Here's how the part is built. I have some questions about the finished solid (model axes, mm). Face numbers are marked on the shaded views. Round coordinates to 2 decimals unless told otherwise and drop trailing zeros. Write each loop counter-clockwise with the first axis right and the second up, starting at its lowest first coordinate (ties: lowest second). Pieces come first, ordered by that corner, then holes. Notation, with made-up numbers: (16, -2.5) -> (43, -2.5) arc R21 ccw to (43, 22.5) -> close; hole circle Ø4 at (34, 87.5). An arc over 180 degrees is marked (long way). Answer in a Markdown table with one row per item.
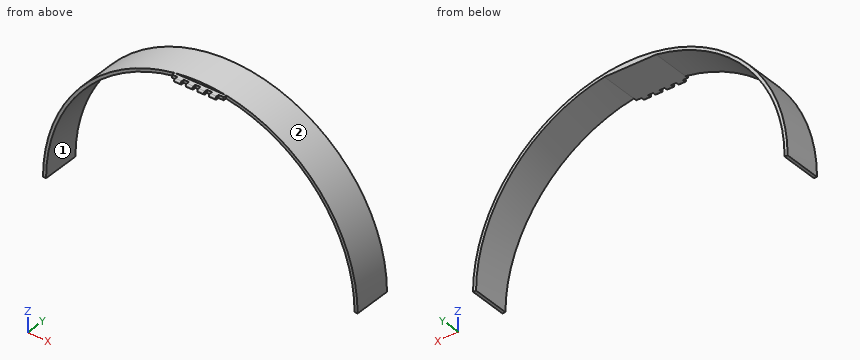
from build123d import *

# Parameters (mm, degrees)
SKETCH1_W              = 50
SKETCH1_H              = 3
BOSS_EXTRUDE1_DEPTH    = 40
SKETCH2_W              = 6.25
SKETCH2_H              = 3
BOSS_EXTRUDE2_DEPTH    = 4
FILLET1_R              = 1.5
LPATTERN1_COUNT        = 4
LPATTERN1_PITCH        = 11.25
FILLET1_OF_LPATTERN1_R = 1.5
SKETCH3_W              = 3
SKETCH3_H              = 37
SKETCH8_R              = 0.75
CUT_EXTRUDE1_DEPTH     = 232.430553417
CUT_EXTRUDE2_DEPTH     = 218.721568988


with BuildPart() as part:
    # Sketch1 → Boss-Extrude1 (new body)
    with BuildSketch(Plane(origin=(0, 0, 0), x_dir=(1, 0, 0), z_dir=(0, 1, 0))):
        Rectangle(SKETCH1_W, SKETCH1_H)
    extrude(amount=BOSS_EXTRUDE1_DEPTH)

    # Sketch2 → Boss-Extrude2 (add)
    with BuildSketch(Plane.XZ):
        with Locations((-16.875, 0)):
            Rectangle(SKETCH2_W, SKETCH2_H)
    boss_extrude2 = extrude(amount=BOSS_EXTRUDE2_DEPTH)

    # Fillet1
    fillet1_edges = [part.edges().sort_by_distance(p)[0] for p in [
        (-16.875, -4, 1.5),
        (-16.875, -4, -1.5),
    ]]
    fillet(fillet1_edges, radius=FILLET1_R - 0.0001)  # a hair under: the kernel refuses the full size

    # LPattern1: Boss-Extrude2 ×4
    with Locations(*[(i * LPATTERN1_PITCH, 0, 0) for i in range(1, LPATTERN1_COUNT)]):
        add(boss_extrude2)

    # Fillet1 of LPattern1
    fillet1_of_lpattern1_edges = [part.edges().sort_by_distance(p)[0] for p in [
        (-5.625, -4, 1.5),
        (-5.625, -4, -1.5),
        (5.625, -4, 1.5),
        (5.625, -4, -1.5),
        (16.875, -4, 1.5),
        (16.875, -4, -1.5),
    ]]
    fillet(fillet1_of_lpattern1_edges, radius=FILLET1_OF_LPATTERN1_R - 0.0001)  # a hair under: the kernel refuses the full size

    # Sweep2: sweep along a path in Sketch7
    with BuildLine(Plane(origin=(0, 38.5, 0), x_dir=(1, 0, 0), z_dir=(0, 1, 0))) as sweep2_path:
        ThreePointArc((-149.86, 148.775138892), (0, -1.084861108), (149.86, 148.775138892))
    # Sketch3 → Sweep2 (sweep)
    with BuildSketch(Plane(origin=(25, 0, 0), x_dir=(0, 0, -1), z_dir=(1, 0, 0))):
        with Locations((0, 21.5)):
            Rectangle(SKETCH3_W, SKETCH3_H)
    sweep(path=sweep2_path.line)

    # Sketch8 → Cut-Extrude1 (cut, through all)
    with BuildSketch(Plane.ZY.offset(20)):
        with Locations((0, -2.5)):
            Circle(SKETCH8_R)
    extrude(amount=-CUT_EXTRUDE1_DEPTH, mode=Mode.SUBTRACT)

    # Sketch9 → Cut-Extrude2 (cut, through all)
    with BuildSketch(Plane(origin=(0, 40, 0), x_dir=(1, 0, 0), z_dir=(0, 1, 0))):
        Polygon((-149.381926595, 148.694252085), (-152.34044383, 148.694252085), (-152.443464298, 148.694252085), (-152.443464298, 149.267987832), align=None)
        Polygon((152.339887493, 148.355558597), (149.339735724, 148.355558597), (149.381926595, 148.856025699), align=None)
    extrude(amount=-CUT_EXTRUDE2_DEPTH, mode=Mode.SUBTRACT)


solid = part.part
1) I want a section at C-C, the plane z = -136. List the corners of the cut face in (x, y) for me, and give its area (3 significant figures).
Response:
| item | result |
|---|---|
| outline | (-151.8, 3) -> (-148.83, 3) -> (-148.83, 40) -> (-151.8, 40) -> close; (148.83, 3) -> (151.8, 3) -> (151.8, 40) -> (148.83, 40) -> close |
| area | 220 mm^2 |
2) For pin 1 (3.5 mm diameter, centred on x = 151, y = 22, fed in from -Z); pin 2 (0.9 mm diameter, centred on y = 2, z = 0, fed in from +X); pin 3 (2.5 mm diameter, centred on y = -1.5, z = 0, fed in from +X); pin 4 (1.2 mm diameter, centred on y = -2.5, z = 0, fed in from +X), each with a flat end and sliding along its axis, tell me the tip position at first contact or that it passes through.
Response:
| item | result |
|---|---|
| pin 1 | stops at z = -148.36 |
| pin 2 | stops at x = 25 |
| pin 3 | stops at x = 20 |
| pin 4 | passes through |
3) I need wall thicknesses on line 1 (Y direction, x = 6, z = 0); line 2 (Z direction, x = -1.5, y = 22.5); line 3 (X direction, y = 20, z = -102). Which ranges of each line are inside material? Lowest first, please. Write a range as [from, to].
Response:
| item | result |
|---|---|
| line 1 | y = [-4, -3.25], [-1.75, 40] |
| line 2 | z = [-1.5, 3.56] |
| line 3 | x = [-144.98, -141.87], [141.87, 144.98] |
4) We'd pull the mould along X, two halves only. Please class the marked faces 1 and 2: +X half, -X half, draft (parallel to the pull), parting line (faces both ways), or undercut.
Response:
| item | result |
|---|---|
| face 1 | undercut |
| face 2 | parting line |
5) I want a section at A-A, the plane z = -97. List the corners of the cut face in (x, y) for me, and give its area (3 significant figures).
Response:
| item | result |
|---|---|
| outline | (-143.27, 3) -> (-140.12, 3) -> (-140.12, 40) -> (-143.27, 40) -> close; (140.12, 3) -> (143.27, 3) -> (143.27, 40) -> (140.12, 40) -> close |
| area | 233 mm^2 |
6) I want a section at D-D, the plane x = 132.5. List the corners of the cut face in (y, z) for me.
Response:
| item | result |
|---|---|
| outline | (3, -79.79) -> (40, -79.79) -> (40, -73.6) -> (3, -73.6) -> close |
